Part model, mm, in its own coordinate system. Face numbers are marked on the shaded views. A direction names the side the tool comes from. Give positions to 0.01 mm unless a question says otherwise; leave off trailing zeros. Write each loop counter-clockwise with the first axis right and the second up, starting at its lowest first coordinate (ties: lowest second). Pieces come first, ordered by that corner, then holes. Notation, with made-up numbers: (31, 85) - (90, 85) arc R9 ccw to (90, 101) - close; hole circle Ø5 at (26.5, 31.25). An arc over 180 degrees is marked (long way). Answer as a JSON object with one key per item and string values. Group by question number.
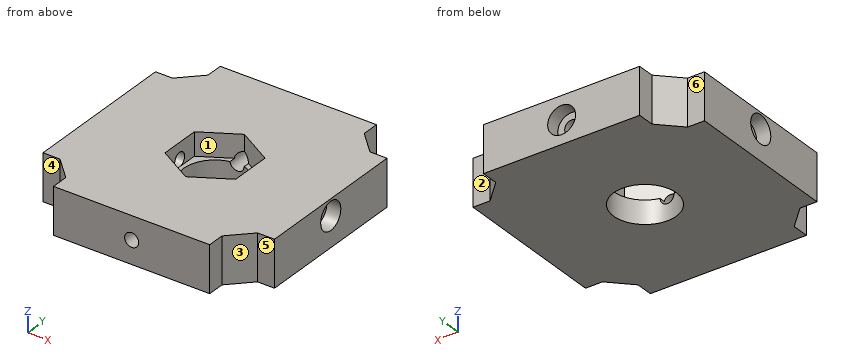
Autodesk Inventor part; units mm, degrees
ref_plane "YZ Plane" through (0, 0, 0) normal (1, 0, 0) x (0, 1, 0)
ref_plane "XZ Plane" through (0, 0, 0) normal (0, 1, 0) x (-1, 0, 0)
ref_plane "XY Plane" through (0, 0, 0) normal (0, 0, 1) x (1, 0, 0)
sketch "草图1" plane through (0, 0, 0) normal (0, 0, 1) x (1, 0, 0)
  line L0 (24.9, 0) -> (24.9, 16.8)
  line L1 (24.9, 0) -> (41.7, 0) construction
  line L2 (24.9, 16.8) -> (21.24, 16.8)
  line L3 (21.24, 16.8) -> (16.7994, 21.2406)
  line L4 (16.7994, 21.2406) -> (16.7994, 24.9006)
  line L5 (16.7994, 24.9006) -> (-0.0006, 24.9006)
  line L6 (-0.0006, 24.9006) -> (-16.8006, 24.9006)
  line L7 (-16.8006, 24.9006) -> (-16.8006, 21.2406)
  line L8 (-16.8006, 21.2406) -> (-21.2413, 16.8)
  line L9 (-21.2413, 16.8) -> (-24.9013, 16.8)
  line L10 (-24.9013, 16.8) -> (-24.9013, 0)
  line L11 (-24.9013, 0) -> (-24.9013, -16.8)
  line L12 (-24.9013, -16.8) -> (-21.2413, -16.8)
  line L13 (-21.2413, -16.8) -> (-16.8006, -21.2406)
  line L14 (-16.8006, -21.2406) -> (-16.8006, -24.9006)
  line L15 (-16.8006, -24.9006) -> (16.7994, -24.9006)
  line L16 (16.7994, -24.9006) -> (16.7994, -21.2406)
  line L17 (16.7994, -21.2406) -> (21.24, -16.8)
  line L18 (21.24, -16.8) -> (24.9, -16.8)
  line L19 (24.9, -16.8) -> (24.9, 0)
  line L20 (-8.7757, 0) -> (-4.3879, 7.6)
  line L21 (-4.3879, 7.6) -> (4.3879, 7.6)
  line L22 (4.3879, 7.6) -> (8.7757, 0)
  line L23 (8.7757, 0) -> (4.3879, -7.6)
  line L24 (4.3879, -7.6) -> (-4.3879, -7.6)
  line L25 (-4.3879, -7.6) -> (-8.7757, 0)
  point P0 (0, 0)
  point P1 (0, 0)
  point P2 (0, 0)
  dimension "d61" = 15.2
extrude "拉伸1" add sketch "草图1" along normal blind 5 and the other way blind 5 contours L19 L18 L17 L16 L15 L14 L13 L12 L11 L10 L9 L8 L7 L6 L5 L4 L3 L2 L0 | L20 L21 L22 L23 L24 L25
sketch "草图2" plane through (0, 0, 5) normal (0, 0, 1) x (1, 0, 0)
  point P0 (0, 0)
sketch "草图3" plane through (0, 0, 5) normal (0, 0, 1) x (1, 0, 0)
  point P0 (0, 0)
sketch "草图4" plane through (0, 0, 5) normal (0, 0, 1) x (1, 0, 0)
  line L0 (7.6, -4.3879) -> (0, -8.7757)
  line L1 (0, -8.7757) -> (-7.6, -4.3879)
  line L2 (-7.6, -4.3879) -> (-7.6, 4.3879)
  line L3 (-7.6, 4.3879) -> (0, 8.7757)
  line L4 (0, 8.7757) -> (7.6, 4.3879)
  line L5 (7.6, 4.3879) -> (7.6, -4.3879)
  point P0 (0, 0)
  point P1 (0, 0)
  dimension "d30" = 15.2
extrude "拉伸2" cut sketch "草图4" against normal blind 5
sketch "草图5" plane through (0, 0, 0) normal (0, 0, 1) x (1, 0, 0)
  point P0 (0, 0)
  point P1 (0, 0)
hole "孔1" at (0, 0, 0) direction (0, 0, -1) diameter 13.5 end through all
sketch "草图6" plane through (-24.9013, -16.8, 5) normal (-1, 0, 0) x (0, 0, 1)
  point P0 (-5, 16.8)
  point P1 (-3.5, 16.8)
hole "孔2" at (-24.9013, 0, 1.5) direction (1, 0, 0) diameter 2.98 end through all counterbore diameter 6 counterbore depth 3
sketch "草图7" plane through (24.9, -16.8, 5) normal (1, 0, 0) x (0, 0, -1)
  point P0 (5, 16.8)
  point P1 (3.5, 16.8)
hole "孔3" at (24.9, 0, 1.5) direction (-1, 0, 0) diameter 2.98 end through all counterbore diameter 6 counterbore depth 3
sketch "草图8" plane through (-16.8006, 24.9006, 5) normal (0, 1, 0) x (1, 0, 0)
  line L0 (24.4006, 5) -> (16.8006, 5)
hole "孔4" at (0, 24.9006, 0) direction (0, -1, 0) diameter 3 end through all counterbore diameter 6 counterbore depth 3
equation "\"d38\" = 厚度"
equation "\"折弯半径\" = 厚度"
equation "\"折弯释压宽度\" = 厚度"
equation "\"折弯释压深度\" = 0.5 * 厚度"
equation "\"拐角释压尺寸\" = 4 * 厚度"
equation "\"最小余量\" = 2 * 厚度"
equation "\"过渡半径\" = 折弯半径"
equation "\"Jacobi半径尺寸\" = 折弯半径"
equation "\"间隙大小\" = 厚度"
properties part number "zhunzhiguan1"
1) Two-plate mould, pull along X, no slides. Class the marked faces 1, 2 and 3: +X half, -X half, draft (parallel to the pull), parting line (faces both ways), or undercut.
2) Saw through at A-A (x = 18). List the corners of the cut face in (y, z).
3) Drop flat-ended pins along their axis: P1, Ø3.5, axis at y = 0, z = 1.5, coming from the +X side; P2, Ø1.8, axis at y = 22.5, z = 1.5, coming from the -X side; P3, Ø1.8, axis at y = 22.5, z = -2, coming from the +X side. Give the stop position or say it passes through.
4) Drill centre lines: line 1 along Y through (x, z) = (-22.9, 1.5); line 2 along Y through (x, z) = (1.5, -2.5); line 3 along X through (y, z) = (3.5, 3.25). Where is each one in solid material? Low to high. Write a range as from..to.
5) Saw through at B-B (x = -5). List the corners of the cut face in (y, z), and give its area (3 significant figures).
6) Which spindle directions (+Z, -Z, +X, -X, +Y, -Y) get a long thin tool onto all of the face, cutting with end or side? Do the marked faces 4, 5 and 6. Say none if no direction does.
Checks:
{
 "1": {"face 1": "undercut", "face 2": "draft", "face 3": "+X half"},
 "2": {"outline": "(-20.04, -5) - (20.04, -5) - (20.04, 5) - (-20.04, 5) - close; hole circle Ø2.98 at (0, 1.5)"},
 "3": {"P1": "x = 21.9", "P2": "x = -16.8", "P3": "x = 16.8"},
 "4": {"line 1": "-16.8..-3, 3..16.8", "line 2": "-24.9..-6.58, 6.58..21.9", "line 3": "-24.9..-7.6, 7.6..24.9"},
 "5": {"outline": "(-24.9, -5) - (-4.53, -5) - (-4.53, 0) - (-5.89, 0) - (-5.89, 5) - (-24.9, 5) - close; (4.53, -5) - (24.9, -5) - (24.9, 5) - (5.89, 5) - (5.89, 0) - (4.53, 0) - close", "area": "394 mm2"},
 "6": {"face 4": "+Z, -Z, -X, -Y", "face 5": "+Z, -Z, +X, -Y", "face 6": "+Z, -Z, -X, +Y"}
}
